Can you work these out from the drawing? Everything is in mm from the part's minimum corner. A direction names the side the tool comes from. Coordinates: 2 decimals unless noted, no trailing zeros. Order: outer loops, then holes, each group sorted by start corner. A loop starts at its lowest first (then second) coordinate and runs counter-clockwise, first axis right, second up. Notation, with made-up numbers: M 24,-28.75 L 60,-28.75 A15 ccw 60,-0.75 Z; hole C 83,1 d2. An arc over 180 degrees is marked long. Answer as a JSON object with one key per item and string values.
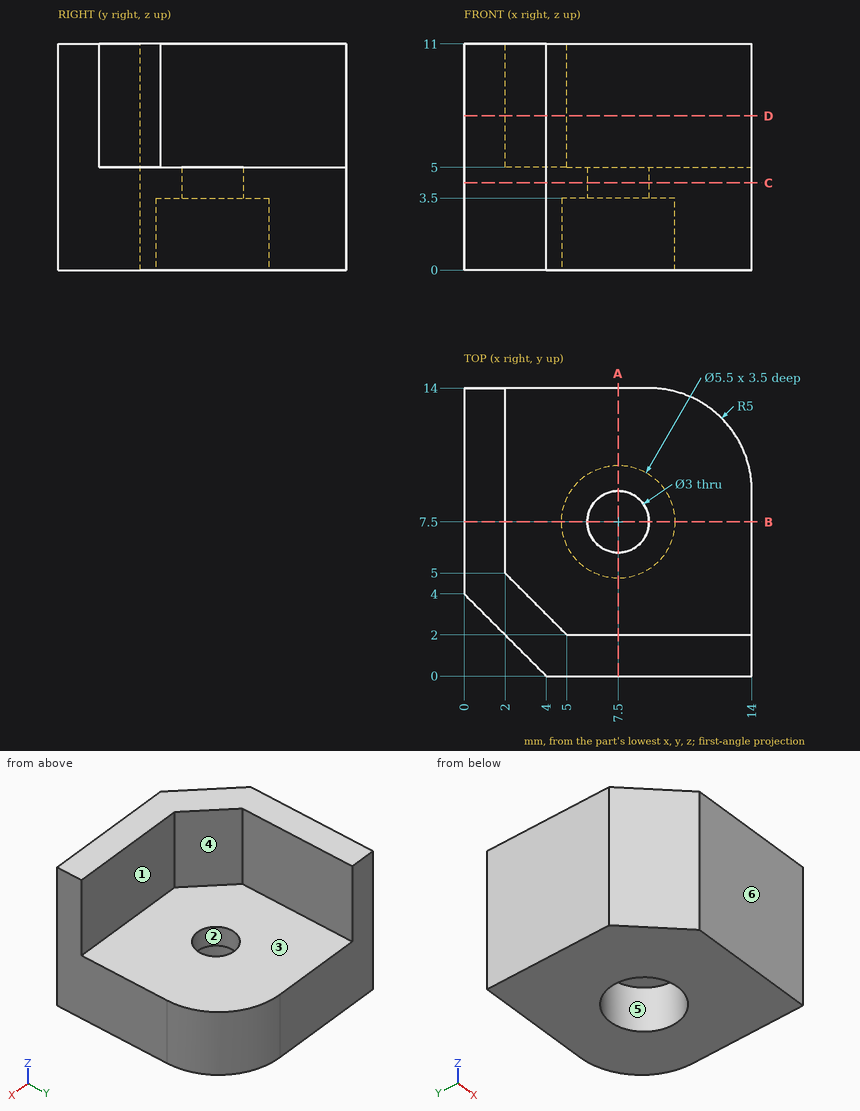
Item 1: Please list where these lines run through material, in increasing order: line 1 (Y direction, x = 7.5, z = 4.4); line 2 (Y direction, x = 7.5, z = 1.9); line 3 (Z direction, x = 6, y = 13.5).
Answers follow:
{"line 1": "y = 0 to 6, 9 to 14", "line 2": "y = 0 to 4.75, 10.25 to 14", "line 3": "z = 0 to 5"}
Item 2: I want a section at A-A, the plane x = 7.5. Write out the boundary of the cut face in (y, z).
Answers follow:
{"outline": "M 0,0 L 4.75,0 L 4.75,3.5 L 6,3.5 L 6,5 L 2,5 L 2,11 L 0,11 Z; M 9,3.5 L 10.25,3.5 L 10.25,0 L 14,0 L 14,5 L 9,5 Z"}
Item 3: I want a section at C-C, the plane z = 4.25. Write out the boundary of the cut face in (x, y), plus the area to 3 significant figures.
Answers follow:
{"outline": "M 0,4 L 4,0 L 14,0 L 14,9 A5 ccw 9,14 L 0,14 Z; hole C 7.5,7.5 d3", "area": "176 mm^2"}
Item 4: If we mould it in two halves opening along Y, with no side actions, what happens to the marked faces 1, 2 and 3? For each: pulls with the +Y half, pulls with the -Y half, needs draft (parallel to the pull), parting line crosses it, or undercut.
Answers follow:
{"face 1": "pulls with the +Y half", "face 2": "undercut", "face 3": "needs draft"}
Item 5: Which directions (+Z, -Z, +X, -X, +Y, -Y) give clear straight access to the entire face, cutting with the end or side of a thin tool? Please do the marked faces 4, 5 and 6.
Answers follow:
{"face 4": "+Z, +X, +Y", "face 5": "-Z", "face 6": "+Z, -Z, +X, -X, -Y"}
Item 6: I'm going to push flat-ended pins straight in: pin 1 (1.8 mm diameter, centred on y = 9, z = 9.5, fed in from +X); pin 2 (4.5 mm diameter, centred on x = 7.5, y = 7.5, fed in from +Z); pin 3 (5 mm diameter, centred on x = 9, z = 9.5, fed in from +Y). Where does each tip first touch, or does it pass through?
Answers follow:
{"pin 1": "stops at x = 2", "pin 2": "stops at z = 5", "pin 3": "stops at y = 2"}
Item 7: I want a section at D-D, the plane z = 7.5. Write out the boundary of the cut face in (x, y).
Answers follow:
{"outline": "M 0,4 L 4,0 L 14,0 L 14,2 L 5,2 L 2,5 L 2,14 L 0,14 Z"}
